from build123d import *

# Parameters (mm, degrees)
F0_W      = 76.2
F0_H      = 76.2
F1_DEPTH  = 2.032
F2_R      = 3.937
F3_DEPTH  = 50.8
F4_W      = 50.8
F4_H      = 50.31309912
F5_DEPTH  = 2.032
F6_W      = 50.8
F6_H      = 50.31309912
F6_W_2    = 45.72
F6_H_2    = 45.72
F7_DEPTH  = 25.4
F8_W      = 50.8
F8_H      = 50.31309912
F8_W_2    = 45.72
F8_H_2    = 45.72
F8_R      = 8.8730231001
F9_DEPTH  = 2.032
F10_W     = 8.89
F10_H     = 11.2548470073
F11_DEPTH = 7.62
F12_R     = 3.937
F13_DEPTH = 50.8
F14_W     = 17.78
F14_H     = 17.78
F15_DEPTH = 2.032
F16_R     = 3.937
F17_DEPTH = 25.4


with BuildPart() as f1:
    # F0 (on Top) → F1 (new body)
    with BuildSketch(Plane.XY):
        Rectangle(F0_W, F0_H)
    extrude(amount=-F1_DEPTH)

    # F2 (on face) → F3 (join)
    with BuildSketch(Plane.XY):
        with Locations((-21.0064100094, -20.9534343708)):
            Circle(F2_R)
        with Locations((-21.0418901269, 20.855767953)):
            Circle(F2_R)
        with Locations((21.0487861186, -21.1718771607)):
            Circle(F2_R)
        with Locations((20.8026003093, 21.1718771607)):
            Circle(F2_R)
    extrude(amount=F3_DEPTH)

    # F4 (on face) → F5 (join)
    with BuildSketch(Plane.XY.offset(50.8)):
        Rectangle(F4_W, F4_H)
    extrude(amount=F5_DEPTH)

    # F6 (on face) → F7 (join)
    with BuildSketch(Plane.XY.offset(52.832)):
        Rectangle(F6_W, F6_H)
        Rectangle(F6_W_2, F6_H_2, mode=Mode.SUBTRACT)
    extrude(amount=F7_DEPTH)

    # F8 (on face) → F9 (join)
    with BuildSketch(Plane.XY.offset(78.232)):
        Rectangle(F8_W, F8_H)
        Rectangle(F8_W_2, F8_H_2, mode=Mode.SUBTRACT)
        Rectangle(F8_W_2, F8_H_2)
        with Locations((-12.8535525873, -10.7279159129)):
            Circle(F8_R, mode=Mode.SUBTRACT)
    extrude(amount=F9_DEPTH)

    # F10 (on face) → F11 (cut)
    with BuildSketch(Plane.XZ.offset(25.15654956)):
        with Locations((16.51, 58.4594235036)):
            Rectangle(F10_W, F10_H)
        with BuildLine():
            ThreePointArc((20.955, 64.0868470073), (16.51, 68.5318470073), (12.065, 64.0868470073))
            Line((12.065, 64.0868470073), (20.955, 64.0868470073))
        make_face()
        with Locations((0, 58.4594235036)):
            Rectangle(F10_W, F10_H)
        with BuildLine():
            ThreePointArc((4.445, 64.0868470073), (0, 68.5318470073), (-4.445, 64.0868470073))
            Line((-4.445, 64.0868470073), (4.445, 64.0868470073))
        make_face()
        with Locations((-16.51, 58.4594235036)):
            Rectangle(F10_W, F10_H)
        with BuildLine():
            ThreePointArc((-12.065, 64.0868470073), (-16.51, 68.5318470073), (-20.955, 64.0868470073))
            Line((-20.955, 64.0868470073), (-12.065, 64.0868470073))
        make_face()
    extrude(amount=-F11_DEPTH, mode=Mode.SUBTRACT)

    # F12 (on face) → F13 (join)
    with BuildSketch(Plane(origin=(0, 0, -2.032), x_dir=(1, 0, 0), z_dir=(0, 0, -1))):
        with Locations((-33.9964929416, 33.9741817005)):
            Circle(F12_R)
        with Locations((34.2564113713, 33.9811018472)):
            Circle(F12_R)
        with Locations((-33.8014231791, -33.7535219774)):
            Circle(F12_R)
        with Locations((33.9347845396, -33.9068524793)):
            Circle(F12_R)
    extrude(amount=F13_DEPTH)

    # F14 (on face) → F15 (join)
    with BuildSketch(Plane(origin=(0, 0, -52.832), x_dir=(1, 0, 0), z_dir=(0, 0, -1))):
        with Locations((-33.9964929416, 33.9741817005)):
            Rectangle(F14_W, F14_H)
        with Locations((34.4249159098, 33.9741817005)):
            Rectangle(F14_W, F14_H)
        with Locations((-33.9227057993, -33.7536521256)):
            Rectangle(F14_W, F14_H)
        with Locations((33.8537693024, -33.9440368116)):
            Rectangle(F14_W, F14_H)
    extrude(amount=F15_DEPTH)

    # F16 (on face) → F17 (join)
    with BuildSketch(Plane.XY.offset(80.264)):
        with Locations((-11.2163906208, 10.1006944331)):
            Circle(F16_R)
        with Locations((9.8858151284, -8.5968601803)):
            Circle(F16_R)
    extrude(amount=F17_DEPTH)


solid = f1.part
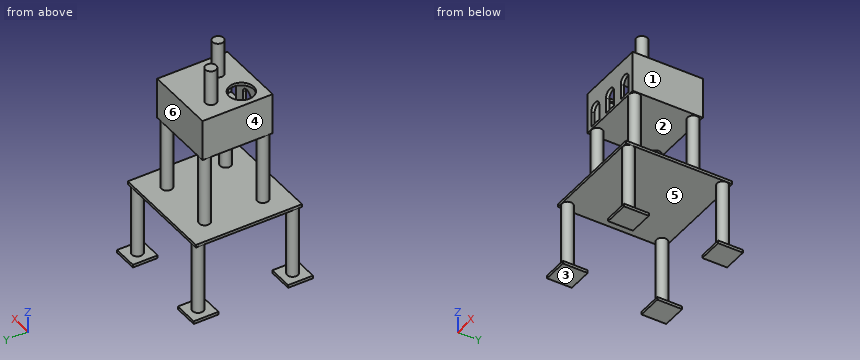
Input: part model. Units: mm. Frame: model coordinates. Face numbers are marked on the shaded views. A direction names the side the tool comes from. Give positions to 0.01 mm unless a question says otherwise; leave off trailing zeros. Order: outer loops, then holes, each group sorted by start corner. A loop starts at its lowest first (then second) coordinate and runs counter-clockwise, first axis right, second up.
Q1. Section A-A on x = 0. Output: boundary loops of the cut face in (y, z).
Checked values:
outline: (-38.1, -2.03) - (38.1, -2.03) - (38.1, 0) - (-38.1, 0) - close; (-25.16, 50.8) - (25.16, 50.8) - (25.16, 80.26) - (-25.16, 80.26) - (-25.16, 68.53) - (-22.86, 68.53) - (-22.86, 78.23) - (22.86, 78.23) - (22.86, 52.83) - (-25.16, 52.83) - close
Q2. Section B-B on z = 2. Output: boundary loops of the cut face in (x, y), and give its area (3 significant figures).
Checked values:
outline: circle Ø7.87 at (-21.04, 20.86); circle Ø7.87 at (-21.01, -20.95); circle Ø7.87 at (20.8, 21.17); circle Ø7.87 at (21.05, -21.17)
area: 195 mm2
Q3. Contact query for flat-ended pins moving along their axis: pin 1 Ø5 at (x, z) = (-7, 59.5) entering from +Y; pin 2 Ø0.6 at (x, z) = (-31.5, -53.5) entering from +Y; pin 3 Ø9 at (x, y) = (-36.5, 35) entering from +Z; pin 4 Ø12 at (x, z) = (17.5, -10.5) entering from -Y. Output: stop coordinate, or through.
Checked values:
pin 1: stops at y = 25.16
pin 2: stops at y = 42.64
pin 3: stops at z = 0
pin 4: passes through
Q4. Draft query along Y for the marked faces 4, 5 and 6. Return one class per face: +Y half, -Y half, draft (parallel to the pull), parting line (faces both ways), or undercut.
Checked values:
face 4: draft
face 5: undercut
face 6: +Y half
Q5. Section C-C on x = -34. Output: boundary loops of the cut face in (y, z), and give its area (3 significant figures).
Checked values:
outline: (-42.86, -54.86) - (-25.08, -54.86) - (-25.08, -52.83) - (-30.04, -52.83) - (-30.04, -2.03) - (29.82, -2.03) - (29.82, -52.83) - (24.86, -52.83) - (24.86, -54.86) - (42.64, -54.86) - (42.64, -52.83) - (37.69, -52.83) - (37.69, -2.03) - (38.1, -2.03) - (38.1, 0) - (-38.1, 0) - (-38.1, -2.03) - (-37.91, -2.03) - (-37.91, -52.83) - (-42.86, -52.83) - close
area: 1,030 mm2
Q6. Set-up query: the marked faces 1, 2 and 3. Return all of +Z, -Z, +X, -X, +Y, -Y with unobstructed straight access to the full face (end or side cutting, diameter ignored); none if empty.
Checked values:
face 1: +Z, +X, +Y, -Y
face 2: none
face 3: -Z, +X, -X, +Y, -Y
Q7. Section D-D on z = 86. Output: boundary loops of the cut face in (x, y).
Checked values:
outline: circle Ø7.87 at (-11.22, 10.1); circle Ø7.87 at (9.89, -8.6)
Q8. Ray query, probe 1 along Z at (x, y) = (-17.5, 10); probe 2 along Z at (x, y) = (21, 17.5); probe 3 along Z at (x, y) = (-9, -10.5). Return the intervals inside material, ascending.
Checked values:
probe 1: z = -2.03 to 0, 50.8 to 52.83, 78.23 to 80.26
probe 2: z = -2.03 to 52.83, 78.23 to 80.26
probe 3: z = -2.03 to 0, 50.8 to 52.83
